Model file for the job. Use its own axes, mm. Coordinates: 2 decimals unless noted, no trailing zeros. Order: outer loops, then holes, each group sorted by start corner. A loop starts at its lowest first (then second) coordinate and runs counter-clockwise, first axis right, second up. Notation, with made-up numbers: M 80,0 L 95,0 A29 cw 95,26 Z; hole C 89,7 d7. An arc over 180 degrees is marked long. Return JSON: item names as keys, results as strings.
```python
from build123d import *

# Parameters (mm, degrees)
REVOLVE1_ANGLE      = 180
SHELL3_T            = -3
BOSS_EXTRUDE1_DEPTH = 5


with BuildPart() as part:
    # Sketch1 → Revolve1 (revolve)
    with BuildSketch(Plane(origin=(0, 0, 0), x_dir=(1, 0, 0), z_dir=(0, 1, 0))):
        with BuildLine():
            Line((-50, 0), (50, 0))
            ThreePointArc((50, 0), (0, 50), (-50, 0))
        make_face()
    revolve(axis=Axis((-50, 0, 0), (1, 0, 0)), revolution_arc=REVOLVE1_ANGLE)

    # Shell3
    shell3_openings = [part.faces().sort_by_distance(p)[0] for p in [
        (0, 0, 0),
    ]]
    offset(amount=SHELL3_T, openings=shell3_openings)

    # Sketch5 → Boss-Extrude1 (add, symmetric)
    with BuildSketch(Plane(origin=(0, 0, 0), x_dir=(0, 0, -1), z_dir=(1, 0, 0))):
        Polygon((-47, 0), (-47, 10), (-137, 10), (-137, 20), (-147, 20), (-147, 0), align=None)
    extrude(amount=BOSS_EXTRUDE1_DEPTH, both=True)


solid = part.part
```
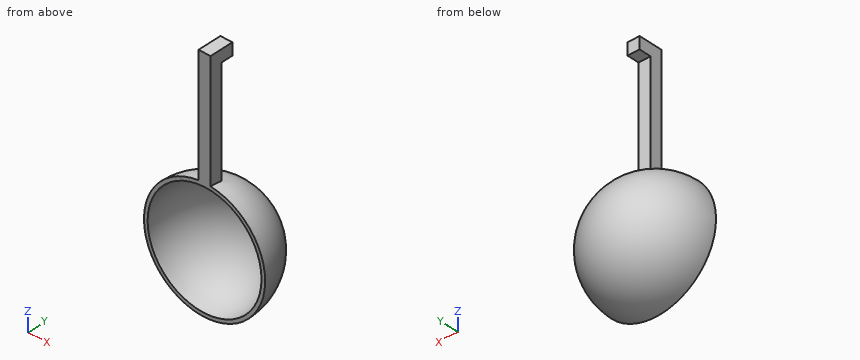
Item 1: Saw through at C-C (y = 24). Write the cut outline in (x, z).
Check result:
{"outline": "C 0,0 d87.73; hole C 0,0 d80.82"}
Item 2: Saw through at A-A (x = -2.5). Write the cut outline in (y, z), and give its area (3 significant figures).
Check result:
{"outline": "M 0,-49.94 A49.94 ccw 10,48.93 L 10,137 L 20,137 L 20,147 L 0,147 L 0,46.93 A46.93 cw 0,-46.93 Z", "area": "1,530 mm2"}
Item 3: Saw through at D-D (x = 40.5). Write the cut outline in (y, z).
Check result:
{"outline": "M 0,-29.32 A29.32 ccw 0,29.32 L 0,23.85 A23.85 cw 0,-23.85 Z"}
Item 4: Wall check: line 1 (Z direction, x = 4.5, y = 11); line 2 (Z direction, x = -0.5, y = 16); line 3 (Z direction, x = -19, y = 30.5). Give the ranges that are in metal, low to high.
Check result:
{"line 1": "z = -48.57 to -45.47, 45.47 to 48.57, 137 to 147", "line 2": "z = -47.37 to -44.19, 44.19 to 47.37, 137 to 147", "line 3": "z = -34.77 to -30.29, 30.29 to 34.77"}
Item 5: Saw through at B-B (z = 111.5). Write the cut outline in (x, y).
Check result:
{"outline": "M -5,0 L 5,0 L 5,10 L -5,10 Z"}
Item 6: Drop flat-ended pins along their axis: pin 1 Ø10 at (y, z) = (6, 119) entering from +X; pin 2 Ø16 at (y, z) = (14.5, 76.5) entering from -X; pin 3 Ø5 at (x, y) = (1, 12.5) entering from -Z; pin 4 Ø2 at (x, z) = (-25, 43.5) entering from -Y. Give the stop position or say it passes through.
Check result:
{"pin 1": "stops at x = 5", "pin 2": "stops at x = -5", "pin 3": "stops at z = -48.98", "pin 4": "stops at y = 0"}
